The listing builds one solid part. Answer for the finished solid, in the listing's coordinates (mm). A direction names the side the tool comes from. Round coordinates to 2 decimals unless told otherwise and drop trailing zeros. Loops run counter-clockwise (first coordinate to the right, second up) from the corner with the lowest first, then second, coordinate; pieces in that order, holes last. Notation, with made-up numbers: (-0.75, -15.75) -> (47.25, -15.75) arc R6 cw to (47.25, -9.75) -> close; hole circle Ø2 at (-1, 32). An arc over 180 degrees is marked (long way). Use a Markdown table: item, result. Add a question column.
Q1. Consider line 1 (Y direction, x = 0, z = 1.75); line 2 (X direction, y = 22, z = 0.5); line 3 (Y direction, x = -4.5, z = 0.7). Determine where each line is inside the solid, lowest interval first.
Q2. Given pin 1 Ø0.9 at (y, z) = (13.5, 1.5) entering from -X; pin 2 Ø1.5 at (y, z) = (-13.5, 2) entering from +X, each flat-ended and moving along its own axis, determine where each tip first touches the part or whether it passes through.
Q3. Section D-D on x = 0 is taken. Give the vertices of the cut face in (y, z), then the cut area to 3 significant figures.
Q4. For a pull along Y with two mould halves and no side action, classify faces 5 (the flat face through (-11, -22, 1)), 6 (the cylindrical face through (16.7, 0.1, 1.5)), 7 (the flat face through (-14, -18, 1)) as released by +Y, released by -Y, zero draft, split by the parting line, or undercut.
Q5. Section A-A on y = 0 is taken. Give the vertices of the cut face in (x, z), then the cut area to 3 significant figures.
Q6. Section C-C on z = 1.95 is taken. Give the vertices of the cut face in (x, y).
Q7. Section B-B on x = 4.5 is taken. Give the vertices of the cut face in (y, z), then the cut area to 3 significant figures.
Q8. Which of the six approach directions +Z, -Z, +X, -X, +Y, -Y give full straight-line access (tool end or side, diameter ignored) to faces 1 (the flat face through (14, 18, 1)), 2 (the flat face through (11, -22, 1)), 3 (the flat face through (14, -18, 1)), 4 (the flat face through (-14, 18, 1))?
from build123d import *

# Parameters (mm, degrees)
CROQUIS1_R              = 11.7
CROQUIS1_W              = 22
CROQUIS1_H              = 2.5
SALIENTE_EXTRUIR1_DEPTH = 3


with BuildPart() as part:
    # Croquis1 → Saliente-Extruir1 (new body)
    with BuildSketch(Plane.XY):
        with BuildLine():
            Line((-14, 9.104394543), (-14, 26.5))
            Line((-14, 26.5), (14, 26.5))
            Line((14, 26.5), (14, 9.104394543))
            ThreePointArc((14, 9.104394543), (16.7, 0), (14, -9.104394543))
            Line((14, -9.104394543), (14, -26.5))
            Line((14, -26.5), (-14, -26.5))
            Line((-14, -26.5), (-14, -9.104394543))
            ThreePointArc((-14, -9.104394543), (-16.7, 0), (-14, 9.104394543))
        make_face()
        Circle(CROQUIS1_R, mode=Mode.SUBTRACT)
        with Locations((0, 22.25)):
            Rectangle(CROQUIS1_W, CROQUIS1_H, mode=Mode.SUBTRACT)
        with Locations((0, -22.25)):
            Rectangle(CROQUIS1_W, CROQUIS1_H, mode=Mode.SUBTRACT)
    extrude(amount=SALIENTE_EXTRUIR1_DEPTH)


solid = part.part
Checked values:
| question | item | result |
|---|---|---|
| 1 | line 1 | y = -26.5 to -23.5, -21 to -11.7, 11.7 to 21, 23.5 to 26.5 |
| 1 | line 2 | x = -14 to -11, 11 to 14 |
| 1 | line 3 | y = -26.5 to -23.5, -21 to -10.8, 10.8 to 21, 23.5 to 26.5 |
| 2 | pin 1 | stops at x = -14 |
| 2 | pin 2 | stops at x = 14 |
| 3 | outline | (-26.5, 0) -> (-23.5, 0) -> (-23.5, 3) -> (-26.5, 3) -> close; (-21, 0) -> (-11.7, 0) -> (-11.7, 3) -> (-21, 3) -> close; (11.7, 0) -> (21, 0) -> (21, 3) -> (11.7, 3) -> close; (23.5, 0) -> (26.5, 0) -> (26.5, 3) -> (23.5, 3) -> close |
| 3 | area | 73.8 mm2 |
| 4 | face 5 | undercut |
| 4 | face 6 | split by the parting line |
| 4 | face 7 | zero draft |
| 5 | outline | (-16.7, 0) -> (-11.7, 0) -> (-11.7, 3) -> (-16.7, 3) -> close; (11.7, 0) -> (16.7, 0) -> (16.7, 3) -> (11.7, 3) -> close |
| 5 | area | 30.0 mm2 |
| 6 | outline | (-14, -26.5) -> (14, -26.5) -> (14, -9.1) arc R16.7 ccw to (14, 9.1) -> (14, 26.5) -> (-14, 26.5) -> (-14, 9.1) arc R16.7 ccw to (-14, -9.1) -> close; hole circle Ø23.4 at (0, 0); hole (-11, -23.5) -> (11, -23.5) -> (11, -21) -> (-11, -21) -> close; hole (-11, 21) -> (11, 21) -> (11, 23.5) -> (-11, 23.5) -> close |
| 7 | outline | (-26.5, 0) -> (-23.5, 0) -> (-23.5, 3) -> (-26.5, 3) -> close; (-21, 0) -> (-10.8, 0) -> (-10.8, 3) -> (-21, 3) -> close; (10.8, 0) -> (21, 0) -> (21, 3) -> (10.8, 3) -> close; (23.5, 0) -> (26.5, 0) -> (26.5, 3) -> (23.5, 3) -> close |
| 7 | area | 79.2 mm2 |
| 8 | face 1 | +Z, -Z, +X, +Y |
| 8 | face 2 | +Z, -Z |
| 8 | face 3 | +Z, -Z, +X, -Y |
| 8 | face 4 | +Z, -Z, -X, +Y |
